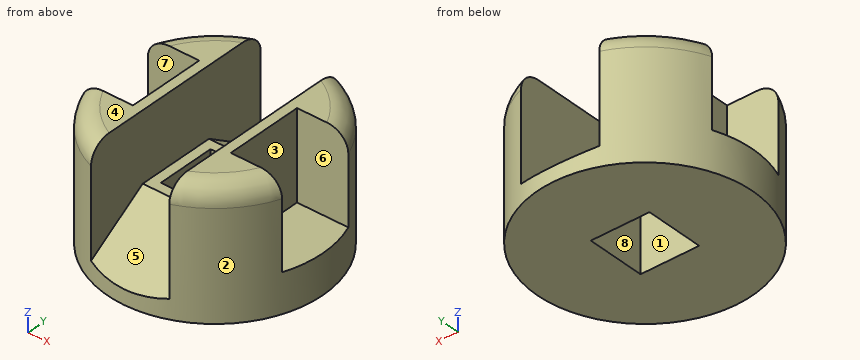
from build123d import *

# Parameters (mm, degrees)
F0_W     = 38.1
F0_H     = 57.15
F2_DEPTH = 25.4
F4_DEPTH = 25.4
F5_W     = 38.1
F5_H     = 38.1
F6_DEPTH = 82.5510001


with BuildPart() as f1:
    # F0 (on Front) → F1 (revolve)
    with BuildSketch(Plane.XZ):
        with BuildLine():
            Line((31.75, 25.4), (69.85, 25.4))
            Line((69.85, 25.4), (69.85, 69.85))
            ThreePointArc((69.85, 69.85), (66.1302561211, 78.8302561211), (57.15, 82.55))
            Line((57.15, 82.55), (31.75, 82.55))
            Line((31.75, 82.55), (31.75, 25.4))
        make_face()
        Polygon((0, 0), (38.1, 0), (69.85, 0), (69.85, 25.4), (31.75, 25.4), (31.75, 82.55), (0, 82.55), align=None)
    revolve(axis=Axis((0, 0, 41.275), (0, 0, -1)))

    # F0 (on Front) → F2 (cut, symmetric)
    with BuildSketch(Plane.XZ):
        with BuildLine():
            Line((31.75, 25.4), (69.85, 25.4))
            Line((69.85, 25.4), (69.85, 69.85))
            ThreePointArc((69.85, 69.85), (66.1302561211, 78.8302561211), (57.15, 82.55))
            Line((57.15, 82.55), (31.75, 82.55))
            Line((31.75, 82.55), (31.75, 25.4))
        make_face()
        with Locations((-50.8, 53.975)):
            Rectangle(F0_W, F0_H)
    extrude(amount=F2_DEPTH, both=True, mode=Mode.SUBTRACT)

    # F3 (on Right) → F4 (cut, symmetric)
    with BuildSketch(Plane.YZ):
        Polygon((69.85, 9.525), (69.85, 82.55), (-69.85, 82.55), (-69.85, 9.525), (-25.4, 38.1), (25.4, 38.1), align=None)
    extrude(amount=F4_DEPTH, both=True, mode=Mode.SUBTRACT)

    # F5 (on face) → F6 (cut, through all)
    with BuildSketch(Plane(origin=(0, 0, 0), x_dir=(1, 0, 0), z_dir=(0, 0, -1))):
        Rectangle(F5_W, F5_H)
    extrude(amount=-F6_DEPTH, mode=Mode.SUBTRACT)


solid = f1.part
CAD build for the part. Positions are in the model's coordinates, mm. Face numbers are marked on the shaded views. A direction names the side the tool comes from. Round coordinates to 2 decimals unless told otherwise and drop trailing zeros. Loops run counter-clockwise (first coordinate to the right, second up) from the corner with the lowest first, then second, coordinate; pieces in that order, holes last. Notation, with made-up numbers: M -26,-16 L -17,-16 A5 ccw -17,-12 Z; hole C 14,17 d9. An arc over 180 degrees is marked long. One line per question, with ' | ' between items. Start each with the question number.
Item 1: Cut at A-A, the plane z = 43.5. Write the cut outline in (x, y), plus the area to 3 significant figures.
Item 2: Cut at D-D, the plane z = 28.5. Write the cut outline in (x, y), plus the area to 3 significant figures.
Item 3: Pin check, flat tips, straight feed: pin 1 Ø6 at (x, z) = (-28, 12.5) entering from -Y; pin 2 Ø6 at (x, y) = (48.5, -2.5) entering from +Z; pin 3 Ø16.5 at (x, z) = (51, 67.5) entering from -Y. Stop position of each tip, or through.
Item 4: Which spindle directions (+Z, -Z, +X, -X, +Y, -Y) get a long thin tool onto all of the face, cutting with end or side? Do the marked faces 5, 6, 7 and 8. Say none if no direction does.
Item 5: Two-plate mould, pull along X, no slides. Class the marked faces 1, 2, 3 and 4: pulls with the +X half, pulls with the -X half, needs draft (parallel to the pull), parting line crosses it, or undercut.
Item 6: Wall check: line 1 (X direction, y = 10, z = 43); line 2 (X direction, y = 4.5, z = 28.5); line 3 (Y direction, x = 45.5, z = 47). Give the ranges that are in metal, low to high.
Item 7: Cut at B-B, the plane x = 0. Write the cut outline in (y, z) (3 decimals).
Item 8: Cut at C-C, the plane y = 0. Write the cut outline in (x, z), plus the area to 3 significant figures.
Responses:
1) outline: M -65.07,-25.4 A69.85 ccw -25.4,-65.07 L -25.4,65.07 A69.85 ccw -65.07,25.4 L -31.75,25.4 L -31.75,-25.4 Z; M 25.4,-65.07 A69.85 ccw 65.07,-25.4 L 31.75,-25.4 L 31.75,25.4 L 65.07,25.4 A69.85 ccw 25.4,65.07 Z | area: 4,680 mm²
2) outline: M -65.07,-25.4 A69.85 ccw -25.4,-65.07 L -25.4,-40.33 L 25.4,-40.33 L 25.4,-65.07 A69.85 ccw 65.07,-25.4 L 31.75,-25.4 L 31.75,25.4 L 65.07,25.4 A69.85 ccw 25.4,65.07 L 25.4,40.33 L -25.4,40.33 L -25.4,65.07 A69.85 ccw -65.07,25.4 L -31.75,25.4 L -31.75,-25.4 Z; hole M -19.05,-19.05 L 19.05,-19.05 L 19.05,19.05 L -19.05,19.05 Z | area: 7,330 mm²
3) pin 1: stops at y = -65.22 | pin 2: stops at z = 25.4 | pin 3: stops at y = -55.24
4) face 5: +Z, -Y | face 6: +Z, +X | face 7: +Z, -X | face 8: +Z, -Z
5) face 1: undercut | face 2: parting line crosses it | face 3: pulls with the +X half | face 4: needs draft
6) line 1: x = -31.75 to -25.4, 25.4 to 31.75 | line 2: x = -31.75 to -19.05, 19.05 to 31.75 | line 3: y = -53 to -25.4, 25.4 to 53
7) outline: M -69.85,0 L -19.05,0 L -19.05,38.1 L -25.4,38.1 L -69.85,9.525 Z; M 19.05,0 L 69.85,0 L 69.85,9.525 L 25.4,38.1 L 19.05,38.1 Z
8) outline: M -69.85,0 L -19.05,0 L -19.05,38.1 L -25.4,38.1 L -25.4,82.55 L -31.75,82.55 L -31.75,25.4 L -69.85,25.4 Z; M 19.05,0 L 69.85,0 L 69.85,25.4 L 31.75,25.4 L 31.75,82.55 L 25.4,82.55 L 25.4,38.1 L 19.05,38.1 Z | area: 3,470 mm²
